Verification items for the finished model (mm, model axes). Face numbers are marked on the shaded views. A direction names the side the tool comes from. Round coordinates to 2 decimals unless told otherwise and drop trailing zeros. Write each loop counter-clockwise with the first axis right and the second up, starting at its lowest first coordinate (ties: lowest second). Pieces come first, ordered by that corner, then holes. Notation, with made-up numbers: (72, -24) -> (98, -24) arc R20 ccw to (98, -18) -> close; hole circle Ø2 at (85.25, -40). An arc over 180 degrees is marked (long way). Use CSV: the item, a comma, the result in double quotes.
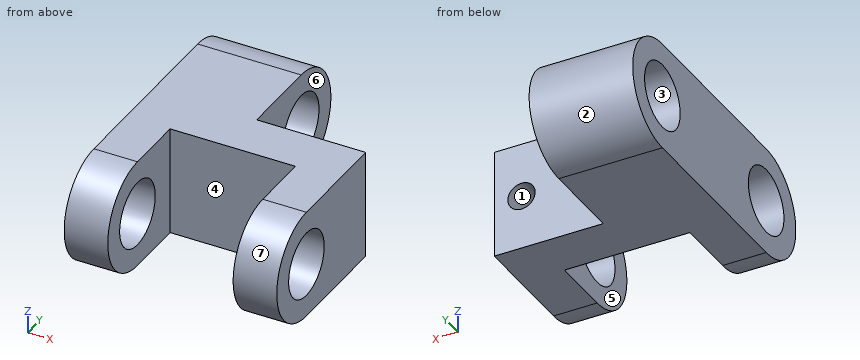
```python
from build123d import *

# Parameters (mm, degrees)
SKETCH_1_R               = 6
EXTRUDE_1_DEPTH          = 39
CUT_EXTRUDE_1_DEPTH      = 49.757050772
CUT_EXTRUDE_1_DEPTH_BACK = 49.757050772
SKETCH_2_W               = 23
SKETCH_2_H               = 34.092407746
CUT_EXTRUDE_2_DEPTH      = 49.757050772
CUT_EXTRUDE_2_DEPTH_BACK = 49.757050772
SKETCH_3_W               = 43.713213687
SKETCH_3_H               = 32.597275916
SKETCH_4_R               = 2.5
CUT_EXTRUDE_3_DEPTH      = 12


with BuildPart() as part:
    # Эскиз1 → Бобышка-Вытянуть1 (new body)
    with BuildSketch(Plane(origin=(0, 0, 0), x_dir=(0, 0, -1), z_dir=(1, 0, 0))):
        with BuildLine():
            Line((10, 17.5), (10, -17.5))
            ThreePointArc((10, -17.5), (0, -27.5), (-10, -17.5))
            Line((-10, -17.5), (-10, 17.5))
            ThreePointArc((-10, 17.5), (0, 27.5), (10, 17.5))
        make_face()
        with Locations((0, 17.5)):
            Circle(SKETCH_1_R, mode=Mode.SUBTRACT)
        with Locations(Location((0, -17.5, 0), (0, 0, 180))):
            Circle(SKETCH_1_R, mode=Mode.SUBTRACT)
    extrude(amount=EXTRUDE_1_DEPTH)

    # Эскиз2 → Вырез-Вытянуть1 (cut, two sides: drawn at the far end of the back side and taken through both)
    with BuildSketch(Plane.XY.offset(-CUT_EXTRUDE_1_DEPTH_BACK)):
        with Locations((19.5, -23.546203873)):
            Rectangle(SKETCH_2_W, SKETCH_2_H)
    extrude(amount=CUT_EXTRUDE_1_DEPTH + CUT_EXTRUDE_1_DEPTH_BACK, mode=Mode.SUBTRACT)

    # Эскиз3 → Вырез-Вытянуть2 (cut, two sides: drawn at the far end of the back side and taken through both)
    with BuildSketch(Plane.XY.offset(-CUT_EXTRUDE_2_DEPTH_BACK)):
        with Locations((40.856606844, 18.798637958)):
            Rectangle(SKETCH_3_W, SKETCH_3_H)
    extrude(amount=CUT_EXTRUDE_2_DEPTH + CUT_EXTRUDE_2_DEPTH_BACK, mode=Mode.SUBTRACT)

    # Эскиз4 → Вырез-Вытянуть3 (cut)
    with BuildSketch(Plane(origin=(0, 2.5, 0), x_dir=(1, 0, 0), z_dir=(0, 1, 0))):
        with Locations(Location((34, 0, 0), (0, 0, 270))):
            Circle(SKETCH_4_R)
    extrude(amount=-CUT_EXTRUDE_3_DEPTH, mode=Mode.SUBTRACT)


solid = part.part
```
Q1. Material ranges on L1, parallel to Y at x = 3, z = 0; L2, parallel to Y at x = 35.5, z = 0; L3, parallel to X at y = -7, z = 1, recorded low to high.
Filled in:
L1,"-27.5 to -23.5, -11.5 to 11.5, 23.5 to 27.5"
L2,"-27.5 to -23.5, -11.5 to -9.5"
L3,"0 to 8, 31 to 31.71, 36.29 to 39"
Q2. Section check C-C (y = 0.5). Record the cut outline in (x, z).
Filled in:
outline,"(0, -10) -> (39, -10) -> (39, 10) -> (0, 10) -> close; hole circle Ø5 at (34, 0)"
Q3. Section check B-B (x = 34). Record the cut outline in (y, z).
Filled in:
outline,"(-17.5, -10) -> (2.5, -10) -> (2.5, -2.5) -> (-9.5, -2.5) -> (-9.5, 2.5) -> (2.5, 2.5) -> (2.5, 10) -> (-17.5, 10) arc R10 ccw to start; hole circle Ø12 at (-17.5, 0)"
Q4. Section check A-A (z = 0). Record the cut outline in (x, y).
Filled in:
outline,"(0, -27.5) -> (8, -27.5) -> (8, -23.5) -> (0, -23.5) -> close; (0, -11.5) -> (8, -11.5) -> (8, -6.5) -> (31, -6.5) -> (31, -11.5) -> (39, -11.5) -> (39, 2.5) -> (36.5, 2.5) -> (36.5, -9.5) -> (31.5, -9.5) -> (31.5, 2.5) -> (19, 2.5) -> (19, 11.5) -> (0, 11.5) -> close; (0, 23.5) -> (19, 23.5) -> (19, 27.5) -> (0, 27.5) -> close; (31, -27.5) -> (39, -27.5) -> (39, -23.5) -> (31, -23.5) -> close"
Q5. Go/stop test with flat-tipped pins: P1, Ø4, axis at x = 34, z = 0, coming from the +Y side; P2, Ø10, axis at x = 23.5, z = -4, coming from the -Y side; P3, Ø1, axis at x = 26.5, z = 1, coming from the +Y side. Record where each tip stops, or that it passes through.
Filled in:
P1,"y = -9.5"
P2,"y = -6.5"
P3,"y = 2.5"
Q6. Mould release check, pull along Y, two halves, no side actions. Record for the marked faces 1, 2, 3 and 4: released by +Y, released by -Y, zero draft, split by the parting line, or undercut.
Filled in:
face 1,"zero draft"
face 2,"released by +Y"
face 3,"undercut"
face 4,"released by -Y"
Q7. Access from +Z, -Z, +X, -X, +Y, -Y to the whole of each face (thin tool, end or side, straight path). Record for the marked faces 5, 6 and 7.
Filled in:
face 5,"+Z, -Z, -Y"
face 6,"+Z, -Z, +X, +Y"
face 7,"+X, -X, -Y"
Q8. Section check D-D (y = -22). Record the cut outline in (x, z).
Filled in:
outline,"(0, -8.93) -> (8, -8.93) -> (8, -3.97) -> (0, -3.97) -> close; (0, 3.97) -> (8, 3.97) -> (8, 8.93) -> (0, 8.93) -> close; (31, -8.93) -> (39, -8.93) -> (39, -3.97) -> (31, -3.97) -> close; (31, 3.97) -> (39, 3.97) -> (39, 8.93) -> (31, 8.93) -> close"
